Geometry check sheet. Reference: drawing and pictorial views, mm from the part's lowest x, y, z. A direction names the side the tool comes from. Round coordinates to 2 decimals unless told otherwise and drop trailing zeros. Write each loop counter-clockwise with the first axis right and the second up, starting at its lowest first coordinate (ties: lowest second). Pieces come first, ordered by that corner, then holes. Notation, with made-up numbers: M -23.75,66.5 L -5.75,66.5 A27 cw -5.75,86.5 Z; hole C 63,26.5 d5. An arc over 180 degrees is marked long. Put each result on its own line as item: value. Start each with the question number.
(1) Section check B-B on x = 41.5. Record the cut outline in (y, z).
(2) Section check D-D on x = 79. Record the cut outline in (y, z).
(3) Section check A-A on z = 6. Record the cut outline in (x, y).
(4) Gauge pin test, flat ends, axial feed: pin 1 (1.4 mm diameter, centred on y = 0.5, z = 3, fed in from +X); pin 2 (0.9 mm diameter, centred on x = 78, y = 1, fed in from -Z); pin 3 (8 mm diameter, centred on x = 65, y = 11, fed in from -Z). Record the tip position at first contact, or that the pin passes through.
(5) Tool access check on the marked faces 1 and 2. Record the directions out of +Z, -Z, +X, -X, +Y, -Y that give a thin tool (end or side, any length) a straight path to the whole face; none if there is none.
(6) Section check C-C on y = 15. Record the cut outline in (x, z).
(7) Material ranges on probe 1 along Y at (x, z) = (17.5, 8); probe 2 along Z at (x, y) = (75, 18.25), recorded low to high.
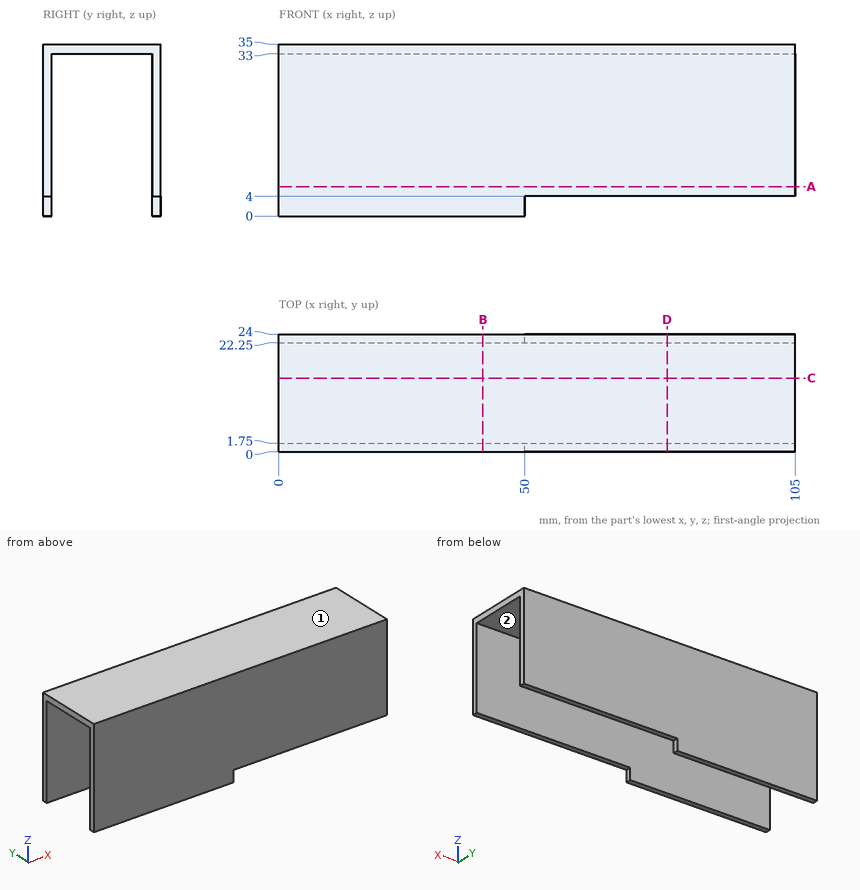
Answers follow:
1. outline: M 0,0 L 1.75,0 L 1.75,33 L 22.25,33 L 22.25,0 L 24,0 L 24,35 L 0,35 Z
2. outline: M 0,4 L 1.75,4 L 1.75,33 L 22.25,33 L 22.25,4 L 24,4 L 24,35 L 0,35 Z
3. outline: M 0,0 L 105,0 L 105,1.75 L 0,1.75 Z; M 0,22.25 L 105,22.25 L 105,24 L 0,24 Z
4. pin 1: stops at x = 50
4. pin 2: stops at z = 4
4. pin 3: stops at z = 33
5. face 1: +Z, +X, -X, +Y, -Y
5. face 2: -Z, +X, -X
6. outline: M 0,33 L 105,33 L 105,35 L 0,35 Z
7. probe 1: y = 0 to 1.75, 22.25 to 24
7. probe 2: z = 33 to 35
